Could you check a few things on this model? Use its own coordinates, in mm. Give positions to 0.01 mm unless a question says otherwise; leave off trailing zeros. Order: outer loops, then holes, each group sorted by start corner. A loop starts at its lowest first (then second) coordinate and runs counter-clockwise, first axis right, second up. Notation, with made-up numbers: (77.5, -2) - (109.5, -2) arc R32 cw to (109.5, 33) - close; hole circle Ø6 at (43.5, -29). An arc over 180 degrees is marked (long way). One line per question, with ' | ' between items. Start each with the question number.
1. Imagine slicing it at B-B (y = -2.75). Please give me the cut outline in (x, z), and give its area (3 significant figures).
2. I need wall thicknesses on probe 1 along Z at (x, y) = (-55, -4); probe 2 along X at (y, z) = (-2.25, 57.5); probe 3 along X at (y, z) = (-4.25, -53). Which ranges of each line are inside material? Lowest first, please. Write a range as from..to.
3. Imagine slicing it at C-C (x = 0). Please give me the cut outline in (y, z), and give its area (3 significant figures).
4. Imagine slicing it at A-A (z = 0). Please give me the cut outline in (x, y).
```python
from build123d import *

# Parameters (mm, degrees)
F0_W     = 150
F0_H     = 150
F0_R     = 3
F0_R_2   = 50
F1_DEPTH = 7
F2_SIZE2 = 5
F2_SIZE  = 5
F3_R     = 5


with BuildPart() as f1:
    # F0 (on Front) → F1 (new body)
    with BuildSketch(Plane.XZ):
        Rectangle(F0_W, F0_H)
        with Locations((-55, -55)):
            Circle(F0_R, mode=Mode.SUBTRACT)
        with Locations((55, -55)):
            Circle(F0_R, mode=Mode.SUBTRACT)
        with Locations((-55, 55)):
            Circle(F0_R, mode=Mode.SUBTRACT)
        Circle(F0_R_2, mode=Mode.SUBTRACT)
        with Locations((55, 55)):
            Circle(F0_R, mode=Mode.SUBTRACT)
    extrude(amount=F1_DEPTH)

    # F2
    f2_edges = [f1.edges().sort_by_distance(p)[0] for p in [
        (-50, 0, 0),
    ]]
    chamfer(f2_edges, length=F2_SIZE, length2=F2_SIZE2)

    # F3
    f3_edges = [f1.edges().sort_by_distance(p)[0] for p in [
        (75, -3.5, 75),
        (-75, -3.5, 75),
        (-75, -3.5, -75),
        (75, -3.5, -75),
    ]]
    fillet(f3_edges, radius=F3_R)


solid = f1.part
```
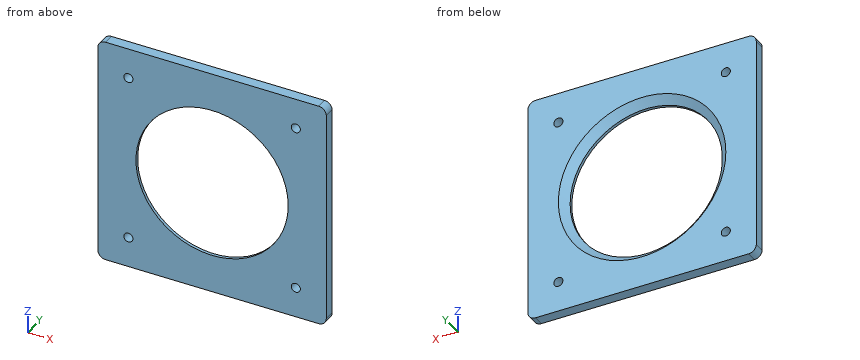
Results found:
1) outline: (-75, -70) arc R5 ccw to (-70, -75) - (70, -75) arc R5 ccw to (75, -70) - (75, 70) arc R5 ccw to (70, 75) - (-70, 75) arc R5 ccw to (-75, 70) - close; hole circle Ø6 at (-55, -55); hole circle Ø6 at (-55, 55); hole circle Ø104.5 at (0, 0); hole circle Ø6 at (55, -55); hole circle Ø6 at (55, 55) | area: 13,800 mm2
2) probe 1: z = -75..-58, -52..52, 58..75 | probe 2: x = -75..-56.66, -53.34..53.34, 56.66..75 | probe 3: x = -75..-57.24, -52.76..52.76, 57.24..75
3) outline: (-7, -75) - (0, -75) - (0, -55) - (-5, -50) - (-7, -50) - close; (-7, 50) - (-5, 50) - (0, 55) - (0, 75) - (-7, 75) - close | area: 325 mm2
4) outline: (-75, -7) - (-50, -7) - (-50, -5) - (-55, 0) - (-75, 0) - close; (50, -7) - (75, -7) - (75, 0) - (55, 0) - (50, -5) - close
